```python
from build123d import *

# Parameters (mm, degrees)
CYLINDER057_R        = 18.5
CYLINDER057_DEPTH    = 10
BOX085108_W          = 40
BOX085108_H          = 11.2
BOX085108_DEPTH      = 40
FILLET005011017060_R = 2


with BuildPart() as cylinder057:
    # Cylinder057 → Cylinder057 (new body)
    with BuildSketch(Plane(origin=(20, 10, 20), x_dir=(1, 0, 0), z_dir=(0, -1, 0))):
        Circle(CYLINDER057_R)
    extrude(amount=CYLINDER057_DEPTH)


with BuildPart() as f_40mm_fan:
    # Box085108 → Box085108 (new body)
    with BuildSketch(Plane.XY):
        with Locations((20, 5.6)):
            Rectangle(BOX085108_W, BOX085108_H)
    extrude(amount=BOX085108_DEPTH)

    # Cut001002016030: cut Cylinder057
    add(cylinder057.part, mode=Mode.SUBTRACT)

    # Fillet005011017060
    fillet005011017060_edges = [f_40mm_fan.edges().sort_by_distance(p)[0] for p in [
        (0, 5.6, 40),
        (0, 5.6, 0),
        (40, 5.6, 40),
        (40, 5.6, 0),
    ]]
    fillet(fillet005011017060_edges, radius=FILLET005011017060_R)


with BuildPart() as f_40mm_fan_1:
    # Fillet005011017060 placement: moved
    add(f_40mm_fan.part.moved(Location((151, 106.8, 6))))


solid = f_40mm_fan_1.part
```
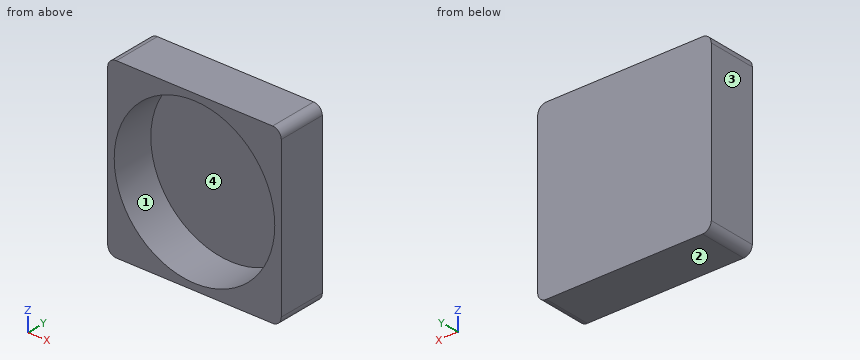
The listing builds one solid part. Answer for the finished solid, in the listing's coordinates (mm). Face numbers are marked on the shaded views. Give positions to 0.01 mm unless a question says otherwise; leave off trailing zeros. Order: outer loops, then holes, each group sorted by start corner. A loop starts at its lowest first (then second) coordinate and runs counter-clockwise, first axis right, second up. Notation, with made-up numbers: M 17,-19.75 L 34,-19.75 A28 ccw 34,13.25 Z; hole C 29,59 d11. An arc over 180 degrees is marked long. Put each result on its own line as item: value. Start each with the question number.
Item 1: The part is cut by section A-A, the plane x = 171. Determine the outline of the cut face in (y, z), and give its area (3 significant figures).
Item 2: For a pull along X with two mould halves and no side action, classify the marked faces 1, 2, 3 and 4 as +X half, -X half, draft (parallel to the pull), parting line (faces both ways), or undercut.
Item 3: Find the intervals of material crossed by line 1 along Z through (x, y) = (171, 110.75); line 2 along Y through (x, z) = (160, 17); line 3 along Z through (x, y) = (179.5, 114), in increasing order.
Item 4: A flat-ended cylindrical pin translates along its axis: P1, Ø3, axis at x = 178.5, z = 13.5, coming from the -Y side. Find the tip coordinate at first contact, or state that the pin passes through.
Item 5: The part is cut by section C-C, the plane z = 26. Determine the outline of the cut face in (x, y).
Item 6: The part is cut by section B-B, the plane y = 108.5. Determine the outline of the cut face in (x, z), and give its area (3 significant figures).
Answer key:
1. outline: M 106.8,6 L 118,6 L 118,46 L 106.8,46 L 106.8,44.5 L 116.8,44.5 L 116.8,7.5 L 106.8,7.5 Z
1. area: 78.0 mm²
2. face 1: undercut
2. face 2: draft
2. face 3: -X half
2. face 4: undercut
3. line 1: z = 6 to 7.5, 44.5 to 46
3. line 2: y = 116.8 to 118
3. line 3: z = 6 to 9.57, 42.43 to 46
4. P1: stops at y = 116.8
5. outline: M 151,106.8 L 152.5,106.8 L 152.5,116.8 L 189.5,116.8 L 189.5,106.8 L 191,106.8 L 191,118 L 151,118 Z
6. outline: M 151,8 A2 ccw 153,6 L 189,6 A2 ccw 191,8 L 191,44 A2 ccw 189,46 L 153,46 A2 ccw 151,44 Z; hole C 171,26 d37
6. area: 521 mm²
